Input: part model. Units: mm. Frame: model coordinates. A direction names the side the tool comes from. Coordinates: 2 decimals unless noted, no trailing zeros. Write each loop counter-clockwise with the first axis right and the second up, starting at its lowest first coordinate (ties: lowest second). Pieces come first, ordered by that corner, then holes. Notation, with made-up numbers: (4.25, 35) -> (39.25, 35) arc R14 ccw to (39.25, 62) -> close; hole circle Ø5 at (71.25, 88.25). An arc over 180 degrees is marked (long way). Use one line per item in the form item = value. Start each with the question number.
(1) Pull-direction query (X, two-part tool) for faces 1 (the face through (0.48, 10.65, 1.19)), 2 (the face through (0, -13, -13.125)), 3 (the face through (-21.095, 4.458, -9.771)); classes: released by +X, released by -X, zero draft, split by the parting line, or undercut.
(2) First-contact query: pin 1 (1.8 mm diameter, centred on x = -22.65, z = -11.275, fed in from +Y); pin 2 (2 mm diameter, centred on x = 14.5, z = -9.5, fed in from +Y); pin 3 (3.5 mm diameter, centred on x = 12.7, z = 0, fed in from +Y); pin 4 (1.2 mm diameter, centred on x = 0.5, z = -0.5, fed in from -Y). Flat tips, straight axial feed; report the tip coordinate or a pass-through.
(3) Cut plane B-B on y = -22.45. Return the cut outline in (x, z) (3 decimals).
(4) Cut plane C-C on x = 2.5. Return the cut outline in (y, z) (3 decimals).
(5) Set-up query: faces 4 (the face through (0, -15, 12.125)), 5 (the face through (11.056, 4.914, -1.048)), 6 (the face through (11.236, 5.766, -0.325)). Return all of +Z, -Z, +X, -X, +Y, -Y with unobstructed straight access to the full face (end or side cutting, diameter ignored); none if empty.
(6) Cut plane A-A on x = 12.7. Return the cut outline in (y, z) (3 decimals), plus the area to 3 significant figures.
(7) Cut plane D-D on y = -15. Return the cut outline in (x, z) (3 decimals).
(8) Ray query, line 1 along Y through (x, z) = (-1, 0); line 2 along X through (y, z) = (8, 0); line 3 along Z through (x, y) = (22.5, -8.5) (3 decimals). Return the intervals inside material, ascending.
```python
from build123d import *

# Parameters (mm, degrees)
SKETCH_1_W               = 49
SKETCH_1_H               = 26.25
EXTRUDE_1_DEPTH          = 5
SKETCH_2_R               = 1.55
CUT_EXTRUDE_1_DEPTH      = 1.1
MIRROR_2_COPY_1_SKETCH_R = 1.55
MIRROR_2_COPY_1_DEPTH    = 1.1
CUT_EXTRUDE_2_DEPTH      = 1.1
SKETCH_4_R               = 1
CUT_EXTRUDE_3_DEPTH      = 50
SKETCH_5_R               = 5
CUT_EXTRUDE_4_DEPTH      = 29.066450167
SKETCH_6_R               = 1.5
SKETCH_6_R_2             = 1
EXTRUDE_2_DEPTH          = 0.5
CUT_EXTRUDE_START        = -1
CUT_EXTRUDE_6_DEPTH      = 1
SKETCH_23_R              = 1.5
CUT_EXTRUDE_14_DEPTH     = 29.066450167
EXTRUDE_START            = 6.5
SKETCH_25_R              = 1.75
SKETCH_25_R_2            = 1.5
EXTRUDE_13_DEPTH         = 6.5
SKETCH_26_R              = 1
EXTRUDE_14_DEPTH         = 15
SKETCH_20_R              = 1.25
SKETCH_20_R_2            = 1
EXTRUDE_10_DEPTH         = 0.5
SKETCH_27_R              = 1.25
SKETCH_27_R_2            = 1
EXTRUDE_15_DEPTH         = 0.5
EXTRUDE_START_2          = 2
SKETCH_28_R              = 1.95
SKETCH_28_R_2            = 1.75
EXTRUDE_16_DEPTH         = 2
SKETCH_30_W              = 49
SKETCH_30_H              = 26.25
EXTRUDE_17_DEPTH         = 32.2
SKETCH_31_R              = 1
CUT_EXTRUDE_15_DEPTH     = 43.536521073
CUT_EXTRUDE_16_REACH     = 62.084
SKETCH_32_R              = 2


with BuildPart() as part:
    # 草图1 → 凸台-拉伸1 (new body)
    with BuildSketch(Plane(origin=(0, 0, 0), x_dir=(1, 0, 0), z_dir=(0, 1, 0))):
        Rectangle(SKETCH_1_W, SKETCH_1_H)
    extrude(amount=EXTRUDE_1_DEPTH)

    # 草图2 → 切除-拉伸1 (cut)
    with BuildSketch(Plane(origin=(0, 5, 0), x_dir=(1, 0, 0), z_dir=(0, 1, 0))):
        with Locations(Location((-22.65, 11.275, 0), (0, 0, 270))):
            Circle(SKETCH_2_R)
    cut_extrude_1 = extrude(amount=-CUT_EXTRUDE_1_DEPTH, mode=Mode.SUBTRACT)

    # 镜向1: 切除-拉伸1 across plane
    add(cut_extrude_1.mirror(Plane(origin=(0, 0, 0), x_dir=(0, 0, 1), z_dir=(1, 0, 0))), mode=Mode.SUBTRACT)

    # 镜向2: 切除-拉伸1 across plane
    add(cut_extrude_1.mirror(Plane.XY), mode=Mode.SUBTRACT)

    # 镜向2 copy 1 sketch → 镜向2 copy 1 (cut)
    with BuildSketch(Plane(origin=(0, 5, 0), x_dir=(-1, 0, 0), z_dir=(0, 1, 0))):
        with Locations(Location((-22.65, 11.275, 0), (0, 0, 270))):
            Circle(MIRROR_2_COPY_1_SKETCH_R)
    extrude(amount=-MIRROR_2_COPY_1_DEPTH, mode=Mode.SUBTRACT)

    # 草图3 → 切除-拉伸2 (cut)
    with BuildSketch(Plane(origin=(0, 5, 0), x_dir=(1, 0, 0), z_dir=(0, 1, 0))):
        with BuildLine():
            Line((-20.705283112, -12.125), (20.705283112, -12.125))
            ThreePointArc((20.705283112, -12.125), (21.120101013, -9.745101013), (23.5, -9.330283112))
            Line((23.5, -9.330283112), (23.5, 9.330283112))
            ThreePointArc((23.5, 9.330283112), (21.120101013, 9.745101013), (20.705283112, 12.125))
            Line((20.705283112, 12.125), (-20.705283112, 12.125))
            ThreePointArc((-20.705283112, 12.125), (-21.120101013, 9.745101013), (-23.5, 9.330283112))
            Line((-23.5, 9.330283112), (-23.5, -9.330283112))
            ThreePointArc((-23.5, -9.330283112), (-21.120101013, -9.745101013), (-20.705283112, -12.125))
        make_face()
    extrude(amount=-CUT_EXTRUDE_2_DEPTH, mode=Mode.SUBTRACT)

    # 草图4 → 切除-拉伸3 (cut)
    with BuildSketch(Plane(origin=(0, 3.9, 0), x_dir=(1, 0, 0), z_dir=(0, 1, 0))):
        with Locations(Location((-22.65, 11.275, 0), (0, 0, 270))):
            Circle(SKETCH_4_R)
        with Locations(Location((22.65, 11.275, 0), (0, 0, 270))):
            Circle(SKETCH_4_R)
        with Locations(Location((22.65, -11.275, 0), (0, 0, 270))):
            Circle(SKETCH_4_R)
        with Locations(Location((-22.65, -11.275, 0), (0, 0, 270))):
            Circle(SKETCH_4_R)
    cut_extrude_3 = extrude(amount=-CUT_EXTRUDE_3_DEPTH, mode=Mode.SUBTRACT)

    # 草图5 → 切除-拉伸4 (cut, through all)
    with BuildSketch(Plane(origin=(0, 3.9, 0), x_dir=(1, 0, 0), z_dir=(0, 1, 0))):
        with Locations(Location((-12.5, 0, 0), (0, 0, 270))):
            Circle(SKETCH_5_R)
    extrude(amount=-CUT_EXTRUDE_4_DEPTH, mode=Mode.SUBTRACT)

    # 草图6 → 凸台-拉伸2 (add)
    with BuildSketch(Plane(origin=(0, 3.9, 0), x_dir=(1, 0, 0), z_dir=(0, 1, 0))):
        with Locations(Location((0.1, 0, 0), (0, 0, 270))):
            Circle(SKETCH_6_R)
        with Locations(Location((0.1, 0, 0), (0, 0, 270))):
            Circle(SKETCH_6_R_2, mode=Mode.SUBTRACT)
    extrude(amount=EXTRUDE_2_DEPTH)

    # 草图10 → 切除-拉伸6 (cut)
    with BuildSketch(Plane.XZ.offset(CUT_EXTRUDE_START)):
        with BuildLine():
            Line((23.5, 9.330283112), (23.5, -9.330283112))
            ThreePointArc((23.5, -9.330283112), (21.120101013, -9.745101013), (20.705283112, -12.125))
            Line((20.705283112, -12.125), (-20.705283112, -12.125))
            ThreePointArc((-20.705283112, -12.125), (-21.120101013, -9.745101013), (-23.5, -9.330283112))
            Line((-23.5, -9.330283112), (-23.5, 9.330283112))
            ThreePointArc((-23.5, 9.330283112), (-21.120101013, 9.745101013), (-20.705283112, 12.125))
            Line((-20.705283112, 12.125), (20.705283112, 12.125))
            ThreePointArc((20.705283112, 12.125), (21.120101013, 9.745101013), (23.5, 9.330283112))
        make_face()
    extrude(amount=CUT_EXTRUDE_6_DEPTH, mode=Mode.SUBTRACT)

    # 草图23 → 切除-拉伸14 (cut, through all)
    with BuildSketch(Plane(origin=(0, 3.9, 0), x_dir=(1, 0, 0), z_dir=(0, 1, 0))):
        with Locations(Location((12.7, 0, 0), (0, 0, 270))):
            Circle(SKETCH_23_R)
    extrude(amount=-CUT_EXTRUDE_14_DEPTH, mode=Mode.SUBTRACT)

    # 草图25 → 凸台-拉伸13 (add)
    with BuildSketch(Plane(origin=(0, 3.9, 0), x_dir=(1, 0, 0), z_dir=(0, 1, 0)).offset(EXTRUDE_START)):
        with Locations(Location((12.7, 0, 0), (0, 0, 90))):
            Circle(SKETCH_25_R)
        with Locations(Location((12.7, 0, 0), (0, 0, 270))):
            Circle(SKETCH_25_R_2, mode=Mode.SUBTRACT)
    extrude(amount=-EXTRUDE_13_DEPTH)

    # 草图26 → 凸台-拉伸14 (add)
    with BuildSketch(Plane(origin=(0, 3.9, 0), x_dir=(1, 0, 0), z_dir=(0, 1, 0))):
        with Locations(Location((0.1, 0, 0), (0, 0, 90))):
            Circle(SKETCH_26_R)
    extrude(amount=EXTRUDE_14_DEPTH)

    # 草图20 → 凸台-拉伸10 (add)
    with BuildSketch(Plane(origin=(0, 10.4, 0), x_dir=(1, 0, 0), z_dir=(0, 1, 0))):
        with Locations(Location((0.1, 0, 0), (0, 0, 270))):
            Circle(SKETCH_20_R)
        with Locations(Location((0.1, 0, 0), (0, 0, 90))):
            Circle(SKETCH_20_R_2, mode=Mode.SUBTRACT)
    extrude(amount=EXTRUDE_10_DEPTH)

    # 草图27 → 凸台-拉伸15 (add)
    with BuildSketch(Plane(origin=(0, 7.4, 0), x_dir=(1, 0, 0), z_dir=(0, 1, 0))):
        with Locations(Location((0.1, 0, 0), (0, 0, 180))):
            Circle(SKETCH_27_R)
        with Locations(Location((0.1, 0, 0), (0, 0, 90))):
            Circle(SKETCH_27_R_2, mode=Mode.SUBTRACT)
    extrude(amount=EXTRUDE_15_DEPTH)

    # 草图28 → 凸台-拉伸16 (add)
    with BuildSketch(Plane(origin=(0, 3.9, 0), x_dir=(1, 0, 0), z_dir=(0, 1, 0)).offset(EXTRUDE_START_2)):
        with Locations(Location((12.7, 0, 0), (0, 0, 90))):
            Circle(SKETCH_28_R)
        with Locations(Location((12.7, 0, 0), (0, 0, 90))):
            Circle(SKETCH_28_R_2, mode=Mode.SUBTRACT)
    extrude(amount=-EXTRUDE_16_DEPTH)

    # 草图30 → 凸台-拉伸17 (add)
    with BuildSketch(Plane.XZ):
        Rectangle(SKETCH_30_W, SKETCH_30_H)
        with BuildLine():
            Line((-20.705283112, 12.125), (20.705283112, 12.125))
            ThreePointArc((20.705283112, 12.125), (21.149262885, 9.774262885), (23.5, 9.330283112))
            Line((23.5, 9.330283112), (23.5, -9.330283112))
            ThreePointArc((23.5, -9.330283112), (21.149262885, -9.774262885), (20.705283112, -12.125))
            Line((20.705283112, -12.125), (-20.705283112, -12.125))
            ThreePointArc((-20.705283112, -12.125), (-21.149262885, -9.774262885), (-23.5, -9.330283112))
            Line((-23.5, -9.330283112), (-23.5, 9.330283112))
            ThreePointArc((-23.5, 9.330283112), (-21.149262885, 9.774262885), (-20.705283112, 12.125))
        make_face(mode=Mode.SUBTRACT)
    extrude(amount=EXTRUDE_17_DEPTH)

    # 草图31 → 切除-拉伸15 (cut, through all)
    with BuildSketch(Plane(origin=(0, 0, 0), x_dir=(1, 0, 0), z_dir=(0, 1, 0))):
        with Locations(Location((22.65, 11.275, 0), (0, 0, 270))):
            Circle(SKETCH_31_R)
    extrude(amount=-CUT_EXTRUDE_15_DEPTH, mode=Mode.SUBTRACT)

    # 镜向3: 切除-拉伸3 across plane
    add(cut_extrude_3.mirror(Plane(origin=(0, 0, 0), x_dir=(0, 0, 1), z_dir=(1, 0, 0))), mode=Mode.SUBTRACT)

    # 草图32 → 切除-拉伸16 (cut, up to next)
    with BuildSketch(Plane(origin=(24.5, 0, 0), x_dir=(0, 0, -1), z_dir=(1, 0, 0)), mode=Mode.PRIVATE) as cut_extrude_16_sk1:
        with Locations((0, -22.45)):
            Circle(SKETCH_32_R)
    cut_extrude_16_tool1 = extrude(cut_extrude_16_sk1.sketch, amount=-CUT_EXTRUDE_16_REACH, mode=Mode.PRIVATE) & part.part
    add(cut_extrude_16_tool1.solids().sort_by_distance((24.5, -22.45, 0))[0], mode=Mode.SUBTRACT)


solid = part.part
```
Values:
q1.face_1 = split by the parting line
q1.face_2 = zero draft
q1.face_3 = undercut
q2.pin_1 = through
q2.pin_2 = 3.9
q2.pin_3 = 10.4
q2.pin_4 = 1
q3.outline = (-24.5, -13.125) -> (24.5, -13.125) -> (24.5, -2) -> (23.5, -2) -> (23.5, -9.33) arc R2.122 ccw to (20.705, -12.125) -> (-20.705, -12.125) arc R2.122 ccw to (-23.5, -9.33) -> (-23.5, 9.33) arc R2.122 ccw to (-20.705, 12.125) -> (20.705, 12.125) arc R2.122 ccw to (23.5, 9.33) -> (23.5, 2) -> (24.5, 2) -> (24.5, 13.125) -> (-24.5, 13.125) -> close; hole circle Ø2 at (-22.65, -11.275); hole circle Ø2 at (-22.65, 11.275); hole circle Ø2 at (22.65, -11.275); hole circle Ø2 at (22.65, 11.275)
q4.outline = (-32.2, -13.125) -> (5, -13.125) -> (5, -12.125) -> (3.9, -12.125) -> (3.9, 12.125) -> (5, 12.125) -> (5, 13.125) -> (-32.2, 13.125) -> (-32.2, 12.125) -> (1, 12.125) -> (1, -12.125) -> (-32.2, -12.125) -> close
q5.face_4 = -Y
q5.face_5 = +Y
q5.face_6 = +Y, -Y
q6.outline = (-32.2, -13.125) -> (5, -13.125) -> (5, -12.125) -> (3.9, -12.125) -> (3.9, -1.95) -> (5.9, -1.95) -> (5.9, -1.75) -> (10.4, -1.75) -> (10.4, -1.5) -> (1, -1.5) -> (1, -12.125) -> (-32.2, -12.125) -> close; (-32.2, 12.125) -> (1, 12.125) -> (1, 1.5) -> (10.4, 1.5) -> (10.4, 1.75) -> (5.9, 1.75) -> (5.9, 1.95) -> (3.9, 1.95) -> (3.9, 12.125) -> (5, 12.125) -> (5, 13.125) -> (-32.2, 13.125) -> close
q6.area = 140 mm2
q7.outline = (-24.5, -13.125) -> (24.5, -13.125) -> (24.5, 13.125) -> (-24.5, 13.125) -> close; hole circle Ø2 at (-22.65, -11.275); hole circle Ø2 at (-22.65, 11.275); hole (-23.5, -9.33) arc R2.122 cw to (-20.705, -12.125) -> (20.705, -12.125) arc R2.122 cw to (23.5, -9.33) -> (23.5, 9.33) arc R2.122 cw to (20.705, 12.125) -> (-20.705, 12.125) arc R2.122 cw to (-23.5, 9.33) -> close; hole circle Ø2 at (22.65, -11.275); hole circle Ø2 at (22.65, 11.275)
q8.line_1 = 1 to 4.4, 7.4 to 7.9, 10.4 to 10.9
q8.line_2 = -0.9 to 1.1, 10.95 to 11.2, 14.2 to 14.45
q8.line_3 = -13.125 to -12.264, -10.286 to -9.158, 9.158 to 10.286, 12.264 to 13.125
